from build123d import *

# Parameters (mm, degrees)
F0_R            = 30.099
F0_R_2          = 23.0124
F1_DEPTH        = 3.048
F3_ANGLE_BACK   = 7.5
F3_ANGLE        = 15
F3_COPIES_COUNT = 3


# Not quite as in the source:
# - a pattern or mirror of a feature is missing from the dataset's text; its kind, count and spacing are read off the source's solid


with BuildPart() as f1:
    # F0 (on Top) → F1 (new body)
    with BuildSketch(Plane.XY):
        Circle(F0_R)
        Circle(F0_R_2, mode=Mode.SUBTRACT)
    extrude(amount=F1_DEPTH)

    # F2 (on Right) → F3 (revolve)
    with BuildSketch(Plane.YZ, mode=Mode.PRIVATE) as f3_sk:
        Polygon((30.099, 6.604), (30.099, 3.048), (30.099, 0), (31.877, 0), (31.877, 8.128), (30.099, 8.128), align=None)
        Polygon((29.718, 6.604), (30.099, 6.604), (30.099, 8.128), align=None)
    f3 = revolve(f3_sk.sketch.rotate(Axis((0, 0, 0), (0, 0, -1)), -F3_ANGLE_BACK), axis=Axis((0, 0, 0), (0, 0, -1)), revolution_arc=F3_ANGLE)

    # F3_copies: F3 ×3 about axis
    f3_copies_axis = Axis((0, 0, 0), (0, 0, 1))
    for i in range(1, F3_COPIES_COUNT):
        add(f3.rotate(f3_copies_axis, i * 360 / F3_COPIES_COUNT))


solid = f1.part
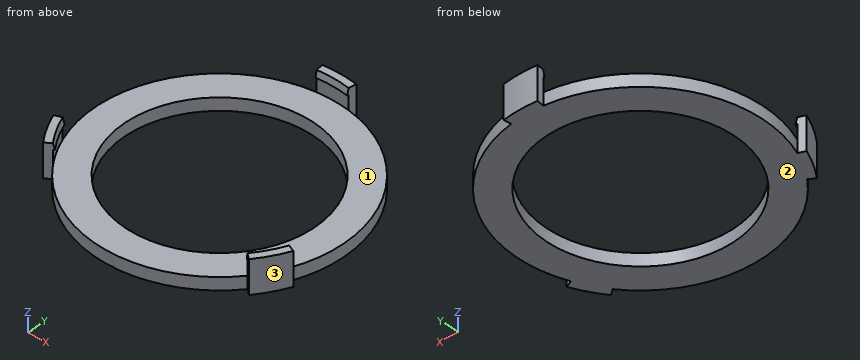
Geometry check sheet. Reference: the model listing, model coordinates, mm. Face numbers are marked on the shaded views. Give positions to 0.01 mm unless a question says otherwise; leave off trailing zeros. Order: outer loops, then holes, each group sorted by start corner. A loop starts at its lowest first (then second) coordinate and runs counter-clockwise, first axis right, second up.
1. Sectioned sample at D-D (x = 0). Record the boundary of the cut face in (y, z), then the cut area to 3 significant figures.
Completed:
outline: (-30.1, 0) - (-23.01, 0) - (-23.01, 3.05) - (-30.1, 3.05) - close; (23.01, 0) - (31.88, 0) - (31.88, 8.13) - (30.1, 8.13) - (29.72, 6.6) - (30.1, 6.6) - (30.1, 3.05) - (23.01, 3.05) - close
area: 57.9 mm2
2. Sectioned sample at A-A (z = 4). Record the boundary of the cut face in (x, y).
Completed:
outline: (-29.45, -12.2) arc R31.88 ccw to (-25.29, -19.41) - (-23.88, -18.32) arc R30.1 cw to (-27.81, -11.52) - close; (-4.16, 31.6) - (-3.93, 29.84) arc R30.1 cw to (3.93, 29.84) - (4.16, 31.6) arc R31.88 ccw to start; (23.88, -18.32) - (25.29, -19.41) arc R31.88 ccw to (29.45, -12.2) - (27.81, -11.52) arc R30.1 cw to start
3. Sectioned sample at B-B (y = 12). Record the boundary of the cut face in (x, z), then the cut area to 3 significant figures.
Completed:
outline: (-27.6, 0) - (-19.64, 0) - (-19.64, 3.05) - (-27.6, 3.05) - close; (19.64, 0) - (27.6, 0) - (27.6, 3.05) - (19.64, 3.05) - close
area: 48.6 mm2
4. Sectioned sample at C-C (x = 21.5). Record the boundary of the cut face in (y, z), then the cut area to 3 significant figures.
Completed:
outline: (-21.06, 0) - (-8.2, 0) - (-8.2, 3.05) - (-21.06, 3.05) - close; (8.2, 0) - (21.06, 0) - (21.06, 3.05) - (8.2, 3.05) - close
area: 78.4 mm2
5. Depth check by flat-ended pin: pin 1 (2 mm diameter, centred on x = 17.5, z = 1, fed in from +Y); pin 2 (1.5 mm diameter, centred on y = -17, z = 6, fed in from +X). Enter the tip coordinate at first touch or a pass-through.
Completed:
pin 1: stops at y = 25.17
pin 2: stops at x = 27.42
6. Draft check along X on the marked faces 1, 2 and 3. Enter one of: pulls with the +X half, pulls with the -X half, needs draft (parallel to the pull), parting line crosses it, or undercut.
Completed:
face 1: undercut
face 2: needs draft
face 3: pulls with the +X half
7. Scan lines: line 1 (Y direction, x = -6, z = 2); line 2 (Z direction, x = -9.5, y = 24); line 3 (Y direction, x = 11, z = 2). Record each from-to range of solid material in increasing order.
Completed:
line 1: y = -29.49 to -22.22, 22.22 to 29.49
line 2: z = 0 to 3.05
line 3: y = -28.02 to -20.21, 20.21 to 28.02
